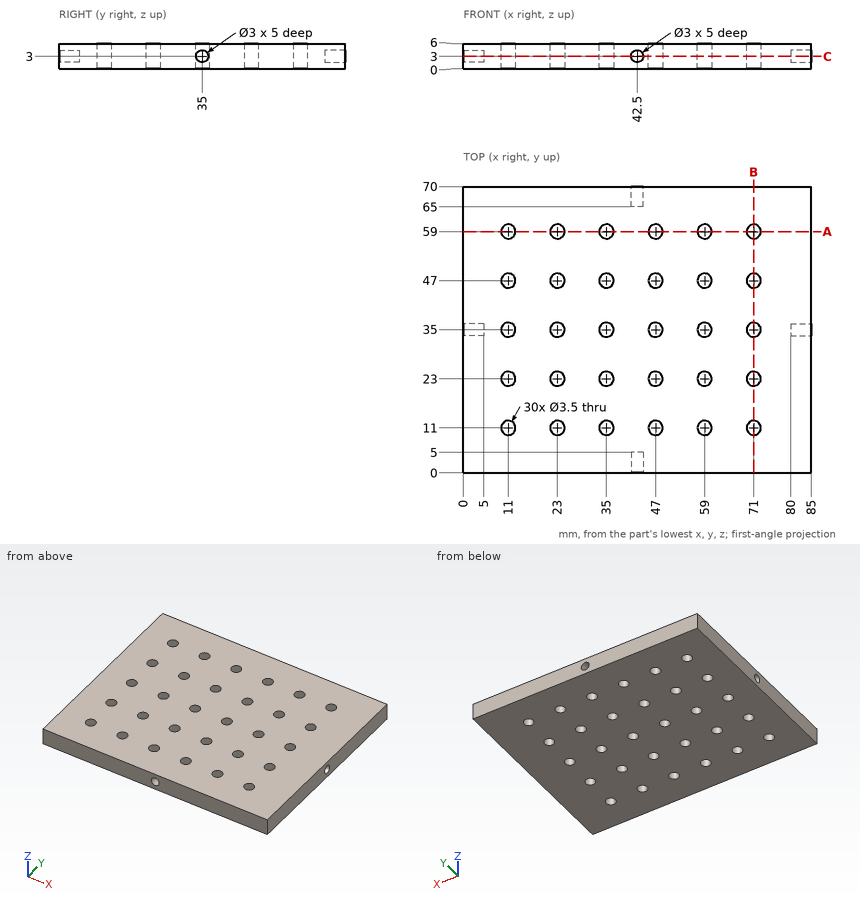
Print and shaded views of the part. All mm, measured from the part's lowest x, y and z. Coordinates: 2 decimals unless noted, no trailing zeros. Loops run counter-clockwise (first coordinate to the right, second up) from the corner with the lowest first, then second, coordinate; pieces in that order, holes last. Notation, with made-up numbers: (73, 3.25) -> (131, 3.25) arc R20 cw to (131, 25.25) -> close; hole circle Ø3 at (-29, 63). An arc over 180 degrees is marked (long way). Use a Markdown table: item, result. Add a question column.
Item 1: Probe probe 1 along Y at (x, z) = (47, 2.05); probe 2 along Y at (x, z) = (72.5, 4.7); probe 3 along Y at (x, z) = (4.5, 2). List the from-to ranges inside material, lowest first.
Item 2: Band-saw the part on C-C on z = 3. Give the number of separate pieces and of enclosed holes in the cut face, plus the area to 3 significant figures.
Item 3: Flat gauge pins, fed straight in: P1, Ø1, axis at y = 23.5, z = 1.5, coming from the -X side; P2, Ø2.5, axis at x = 42.5, z = 3, coming from the +Y side. Where does each tip first touch, or does it go through?
Item 4: Band-saw the part on B-B on x = 71. Write the cut outline in (y, z).
Item 5: Band-saw the part on A-A on y = 59. Write the cut outline in (x, z), plus the area to 3 significant figures.
Geometry says:
| question | item | result |
|---|---|---|
| 1 | probe 1 | 0 to 9.25, 12.75 to 21.25, 24.75 to 33.25, 36.75 to 45.25, 48.75 to 57.25, 60.75 to 70 |
| 1 | probe 2 | 0 to 10.1, 11.9 to 22.1, 23.9 to 34.1, 35.9 to 46.1, 47.9 to 58.1, 59.9 to 70 |
| 1 | probe 3 | 0 to 33.88, 36.12 to 70 |
| 2 | separate pieces | 1 |
| 2 | enclosed holes | 30 |
| 2 | area | 5,600 mm² |
| 3 | P1 | x = 0 |
| 3 | P2 | y = 65 |
| 4 | outline | (0, 0) -> (9.25, 0) -> (9.25, 6) -> (0, 6) -> close; (12.75, 0) -> (21.25, 0) -> (21.25, 6) -> (12.75, 6) -> close; (24.75, 0) -> (33.25, 0) -> (33.25, 6) -> (24.75, 6) -> close; (36.75, 0) -> (45.25, 0) -> (45.25, 6) -> (36.75, 6) -> close; (48.75, 0) -> (57.25, 0) -> (57.25, 6) -> (48.75, 6) -> close; (60.75, 0) -> (70, 0) -> (70, 6) -> (60.75, 6) -> close |
| 5 | outline | (0, 0) -> (9.25, 0) -> (9.25, 6) -> (0, 6) -> close; (12.75, 0) -> (21.25, 0) -> (21.25, 6) -> (12.75, 6) -> close; (24.75, 0) -> (33.25, 0) -> (33.25, 6) -> (24.75, 6) -> close; (36.75, 0) -> (45.25, 0) -> (45.25, 6) -> (36.75, 6) -> close; (48.75, 0) -> (57.25, 0) -> (57.25, 6) -> (48.75, 6) -> close; (60.75, 0) -> (69.25, 0) -> (69.25, 6) -> (60.75, 6) -> close; (72.75, 0) -> (85, 0) -> (85, 6) -> (72.75, 6) -> close |
| 5 | area | 384 mm² |
